Geometry check sheet. Reference: the model listing, model coordinates, mm. A direction names the side the tool comes from. Coordinates: 2 decimals unless noted, no trailing zeros. Loops run counter-clockwise (first coordinate to the right, second up) from the corner with the lowest first, then second, coordinate; pieces in that order, holes last. Notation, with made-up numbers: (57, 50) -> (105, 50) arc R34 ccw to (105, 89) -> close; hole circle Ø10 at (-34.5, 89.25). An arc over 180 degrees is marked (long way). Answer as a JSON object with one key per item and string values.
from build123d import *

# Parameters (mm, degrees)
SKETCH3_W                   = 20
SKETCH3_H                   = 40
SKETCH3_W_2                 = 16
SKETCH3_H_2                 = 36
BASE_FLANGE1_DEPTH          = 500
TAP_DRILL_FOR_M6X1_0_TAP1_D = 5


# Sheet-metal steps are written as plain solids
with BuildPart() as part:
    # Sketch3 → Base-Flange1 (new body)
    with BuildSketch(Plane(origin=(0, 0, 0), x_dir=(1, 0, 0), z_dir=(0, 1, 0))):
        Rectangle(SKETCH3_W, SKETCH3_H)
        Rectangle(SKETCH3_W_2, SKETCH3_H_2, mode=Mode.SUBTRACT)
    extrude(amount=-BASE_FLANGE1_DEPTH)

    # Tap Drill for M6x1.0 Tap1 (through all)
    with Locations(Plane(origin=(10, 0, 0), x_dir=(0, 0, -1), z_dir=(1, 0, 0))):
        with Locations((-12, -484), (12, -484)):
            Hole(TAP_DRILL_FOR_M6X1_0_TAP1_D / 2)


solid = part.part
1. Thickness scan on probe 1 along Z at (x, y) = (-8.75, -484); probe 2 along X at (y, z) = (-102.5, 16); probe 3 along Z at (x, y) = (1.5, -183). Record the ranges inside material, lowest first. Write a range as from..to.
Evaluation:
{"probe 1": "z = -20..-14.5, -9.5..9.5, 14.5..20", "probe 2": "x = -10..-8, 8..10", "probe 3": "z = -20..-18, 18..20"}
2. Mould release check, pull along X, two halves, no side actions. Record for faces 1 (the face through (-8, -246, 0)), 2 (the face through (-10, -246, 0)), 3 (the face through (-8.2, -500, -1.6)): released by +X, released by -X, zero draft, split by the parting line, or undercut.
Evaluation:
{"face 1": "undercut", "face 2": "released by -X", "face 3": "zero draft"}
3. Section check A-A, the plane y = -330. Record the boundary of the cut face in (x, z).
Evaluation:
{"outline": "(-10, -20) -> (10, -20) -> (10, 20) -> (-10, 20) -> close; hole (-8, -18) -> (8, -18) -> (8, 18) -> (-8, 18) -> close"}
4. Tool access check on faces 4 (the face through (8, -246, 0)), 5 (the face through (-8.2, 0, -1.6)). Record the directions out of +Z, -Z, +X, -X, +Y, -Y that give a thin tool (end or side, any length) a straight path to the whole face; none if there is none.
Evaluation:
{"face 4": "+Y, -Y", "face 5": "+Z, -Z, +X, -X, +Y"}
5. Section check B-B, the plane x = 1. Record the boundary of the cut face in (y, z).
Evaluation:
{"outline": "(-500, -20) -> (0, -20) -> (0, -18) -> (-500, -18) -> close; (-500, 18) -> (0, 18) -> (0, 20) -> (-500, 20) -> close"}
